For this review, take the finished solid that the model builds, in its own axes (mm). Face numbers are marked on the shaded views. A direction names the side the tool comes from. Round coordinates to 2 decimals unless told otherwise and drop trailing zeros. Loops run counter-clockwise (first coordinate to the right, second up) from the corner with the lowest first, then second, coordinate; pieces in that order, holes last. Notation, with made-up numbers: (84, 64.25) -> (93, 64.25) arc R25 cw to (93, 81.25) -> close; hole circle Ø7 at (-38, 6). An arc over 180 degrees is marked (long way). Write each question's results on one line, items separated by ' | '.
```python
from build123d import *

# Parameters (mm, degrees)
BOX050_W               = 25
BOX050_H               = 16
BOX050_DEPTH           = 15
BOX048_W               = 25
BOX048_H               = 24
BOX048_DEPTH           = 2
BOX043_W               = 20
BOX043_H               = 5
BOX043_DEPTH           = 12
CYLINDER020_R          = 1.7
CYLINDER020_DEPTH      = 30
CYLINDER020_ROLL_ANGLE = 90
BOX047_W               = 20
BOX047_H               = 2
BOX047_DEPTH           = 26
BOX046_W               = 20
BOX046_H               = 2
BOX046_DEPTH           = 26
BOX045_W               = 20
BOX045_H               = 5
BOX045_DEPTH           = 12
BOX044_W               = 20
BOX044_H               = 5
BOX044_DEPTH           = 12
BOX049_W               = 25
BOX049_H               = 16
BOX049_DEPTH           = 15


with BuildPart() as cube025:
    # Box050 → Box050 (new body)
    with BuildSketch(Plane(origin=(-24, -8, 11), x_dir=(1, 0, 0), z_dir=(0, 0, 1))):
        with Locations((12.5, 8)):
            Rectangle(BOX050_W, BOX050_H)
    extrude(amount=BOX050_DEPTH)


with BuildPart() as cube023:
    # Box048 → Box048 (new body)
    with BuildSketch(Plane(origin=(-34.5, -12, 25), x_dir=(1, 0, 0), z_dir=(0, 0, 1))):
        with Locations((12.5, 12)):
            Rectangle(BOX048_W, BOX048_H)
    extrude(amount=BOX048_DEPTH)


with BuildPart() as cube018:
    # Box043 → Box043 (new body)
    with BuildSketch(Plane(origin=(-37.5, -2.5, 14), x_dir=(1, 0, 0), z_dir=(0, 0, 1))):
        with Locations((10, 2.5)):
            Rectangle(BOX043_W, BOX043_H)
    extrude(amount=BOX043_DEPTH)


with BuildPart() as fusion009:
    # Cylinder020 → Cylinder020 (new body)
    with BuildSketch(Plane.XY):
        Circle(CYLINDER020_R)
    extrude(amount=CYLINDER020_DEPTH)


with BuildPart() as fusion009_1:
    # Cylinder020 roll: moved
    add(fusion009.part.rotate(Axis((0, 0, 0), (1, 0, 0)), CYLINDER020_ROLL_ANGLE))


with BuildPart() as fusion009_2:
    # Cylinder020 placement: moved
    add(fusion009_1.part.moved(Location((-27.5, 16, 20))))

    # Fusion009: union Cube018
    add(cube018.part)


with BuildPart() as fusion010:
    # Box047 → Box047 (new body)
    with BuildSketch(Plane(origin=(-32.5, 7, 0), x_dir=(1, 0, 0), z_dir=(0, 0, 1))):
        with Locations((10, 1)):
            Rectangle(BOX047_W, BOX047_H)
    extrude(amount=BOX047_DEPTH)

    # Fusion010: union Fusion009
    add(fusion009_2.part)


with BuildPart() as fusion011:
    # Box046 → Box046 (new body)
    with BuildSketch(Plane(origin=(-32.5, -9, 0), x_dir=(1, 0, 0), z_dir=(0, 0, 1))):
        with Locations((10, 1)):
            Rectangle(BOX046_W, BOX046_H)
    extrude(amount=BOX046_DEPTH)

    # Fusion011: union Fusion010
    add(fusion010.part)


with BuildPart() as fusion012:
    # Box045 → Box045 (new body)
    with BuildSketch(Plane(origin=(-42.5, 7, 14), x_dir=(1, 0, 0), z_dir=(0, 0, 1))):
        with Locations((10, 2.5)):
            Rectangle(BOX045_W, BOX045_H)
    extrude(amount=BOX045_DEPTH)

    # Fusion012: union Fusion011
    add(fusion011.part)


with BuildPart() as fusion014:
    # Box044 → Box044 (new body)
    with BuildSketch(Plane(origin=(-42.5, -12, 14), x_dir=(1, 0, 0), z_dir=(0, 0, 1))):
        with Locations((10, 2.5)):
            Rectangle(BOX044_W, BOX044_H)
    extrude(amount=BOX044_DEPTH)

    # Fusion013: union Fusion012
    add(fusion012.part)

    # Fusion014: union Cube023
    add(cube023.part)


with BuildPart() as fusion016:
    # Box049 → Box049 (new body)
    with BuildSketch(Plane(origin=(-26, -8, 0), x_dir=(1, 0, 0), z_dir=(0, 0, 1))):
        with Locations((12.5, 8)):
            Rectangle(BOX049_W, BOX049_H)
    extrude(amount=BOX049_DEPTH)

    # Fusion015: union Fusion014
    add(fusion014.part)

    # Fusion016: union Cube025
    add(cube025.part)


solid = fusion016.part
```
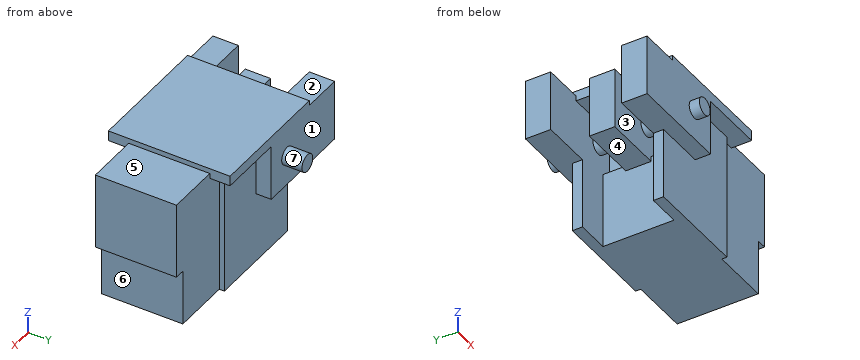
1. For pin 1 (11 mm diameter, centred on x = -5.5, z = 13, fed in from -Y); pin 2 (12 mm diameter, centred on y = 5.5, z = 4.5, fed in from +X); pin 3 (5 mm diameter, centred on x = -1.5, y = 0.5, fed in from +Z), all flat-tipped, find the tip position at first contact; note any pin that passes through.
Values found:
pin 1: stops at y = -8 | pin 2: stops at x = -1 | pin 3: stops at z = 26
2. To check wall thickness, follow probe 1 along Y at (x, z) = (-28, 16); probe 2 along Y at (x, z) = (-31, 9); probe 3 along Z at (x, y) = (-17.5, 11.25). State the ranges of each line that lie inside material, in increasing order.
Values found:
probe 1: y = -12 to -7, -2.5 to 2.5, 7 to 12 | probe 2: y = -9 to -7, 7 to 9 | probe 3: z = 25 to 27
3. Consider section B-B (y = -3.5). State the section outline as (x, z) points.
Values found:
outline: (-34.5, 25) -> (-24, 25) -> (-24, 15) -> (-26, 15) -> (-26, 0) -> (-1, 0) -> (-1, 11) -> (1, 11) -> (1, 26) -> (-9.5, 26) -> (-9.5, 27) -> (-34.5, 27) -> close; circle Ø3.4 at (-27.5, 20)
4. Tool access review of the marked faces 4, 5, 6 and 7: name each direction out of +Z, -Z, +X, -X, +Y, -Y from which nothing blocks a thin tool from reaching the whole face with its end or side.
Values found:
face 4: -Z, -X | face 5: +Z, +X, +Y, -Y | face 6: -Z, +X, +Y, -Y | face 7: +Y
5. Consider section A-A (x = -27.5). Give the number of separate pieces and of enclosed holes in the cut face, plus the area to 3 significant figures.
Values found:
separate pieces: 1 | enclosed holes: 2 | area: 320 mm2
6. Draft analysis for pull direction Y (two halves, no side actions). For the marked faces 1, 2 and 3, state which applies: released by +Y, released by -Y, zero draft, split by the parting line, or undercut.
Values found:
face 1: released by +Y | face 2: zero draft | face 3: undercut
7. Consider section D-D (z = 16). State the section outline as (x, y) points, plus the area to 4 significant figures.
Values found:
outline: (-42.5, -12) -> (-22.5, -12) -> (-22.5, -9) -> (-12.5, -9) -> (-12.5, -8) -> (1, -8) -> (1, 8) -> (-12.5, 8) -> (-12.5, 9) -> (-22.5, 9) -> (-22.5, 12) -> (-42.5, 12) -> (-42.5, 7) -> (-24, 7) -> (-24, 2.5) -> (-37.5, 2.5) -> (-37.5, -2.5) -> (-24, -2.5) -> (-24, -7) -> (-42.5, -7) -> close | area: 684.5 mm2
8. Consider section C-C (x = -38). State the section outline as (y, z) points.
Values found:
outline: (-12, 14) -> (-7, 14) -> (-7, 26) -> (-12, 26) -> close; (7, 14) -> (12, 14) -> (12, 26) -> (7, 26) -> close
